```python
from build123d import *

# Parameters (mm, degrees)
SKETCH1_R           = 5
SKETCH1_R_2         = 2.55
BOSS_EXTRUDE1_DEPTH = 6
CHAMFER1_SIZE       = 0.2


with BuildPart() as part:
    # Sketch1 → Boss-Extrude1 (new body)
    with BuildSketch(Plane.XY):
        Circle(SKETCH1_R)
        Circle(SKETCH1_R_2, mode=Mode.SUBTRACT)
    extrude(amount=BOSS_EXTRUDE1_DEPTH)

    # Chamfer1
    chamfer1_edges = [part.edges().sort_by_distance(p)[0] for p in [
        (-5, 0, 0),
        (-5, 0, 6),
        (-2.55, 0, 0),
        (-2.55, 0, 6),
    ]]
    chamfer(chamfer1_edges, length=CHAMFER1_SIZE)


solid = part.part
```
Part model, mm, in its own coordinate system. Round coordinates to 2 decimals unless told otherwise and drop trailing zeros. Loops run counter-clockwise (first coordinate to the right, second up) from the corner with the lowest first, then second, coordinate; pieces in that order, holes last.
Item 1: Cut at A-A, the plane x = 0. Give the cut face in (y, z).
Item 2: Mould opens along X. For faces 1 (the face through (-1.08, -4.88, 2.96)), 2 (the face through (1.18, -2.26, 2.96)), 3 (the face through (2.1, -2.1, 6)) say: +X half, -X half, draft (parallel to the pull), parting line (faces both ways), or undercut.
Item 3: Cut at C-C, the plane z = 2.2. Give the cut face in (x, y).
Item 4: Drill centre lines: line 1 (Y direction, x = 0, z = 4.3); line 2 (X direction, y = -0.25, z = 0.75); line 3 (Y direction, x = -1.75, z = 2.85). Where is each one in solid material? Low to high.
Item 5: Drop flat-ended pins along their axis: P1, Ø1.5, axis at x = -2, z = 1, coming from the -Y side; P2, Ø1, axis at y = 2.5, z = 2, coming from the -X side. Give the stop position or say it passes through.
A:
1. outline: (-5, 0.2) - (-4.8, 0) - (-2.75, 0) - (-2.55, 0.2) - (-2.55, 5.8) - (-2.75, 6) - (-4.8, 6) - (-5, 5.8) - close; (2.55, 0.2) - (2.75, 0) - (4.8, 0) - (5, 0.2) - (5, 5.8) - (4.8, 6) - (2.75, 6) - (2.55, 5.8) - close
2. face 1: parting line
2. face 2: undercut
2. face 3: draft
3. outline: circle Ø10 at (0, 0); hole circle Ø5.1 at (0, 0)
4. line 1: y = -5 to -2.55, 2.55 to 5
4. line 2: x = -4.99 to -2.54, 2.54 to 4.99
4. line 3: y = -4.68 to -1.85, 1.85 to 4.68
5. P1: stops at y = -4.84
5. P2: stops at x = -4.58
